Can you work these out from the model? Positions are in its coordinate system, mm. Round coordinates to 2 decimals unless told otherwise and drop trailing zeros. Write each loop counter-clockwise with the first axis right and the second up, starting at its lowest first coordinate (ties: lowest second). Pieces come first, ordered by that corner, then holes. Notation, with made-up numbers: (31, -25) -> (86, -25) arc R13 cw to (86, 0) -> close; hole circle Ø2 at (18.5, 13). An arc over 180 degrees is marked (long way). Use CSV: the item, a comma, the result in double quotes.
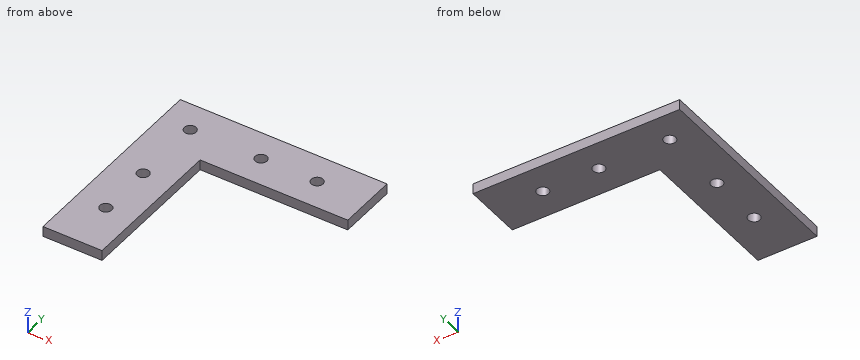
```python
from build123d import *

# Parameters (mm, degrees)
F0_R     = 2
F1_DEPTH = 3.5


with BuildPart() as f1:
    # F0 (on Top) → F1 (new body)
    with BuildSketch(Plane.XY):
        Polygon((-10, -10), (-10, -60), (10, -60), (10, -10), (60, -10), (60, 10), (10, 10), (-10, 10), align=None)
        with Locations((0, -43)):
            Circle(F0_R, mode=Mode.SUBTRACT)
        with Locations((0, -24)):
            Circle(F0_R, mode=Mode.SUBTRACT)
        Circle(F0_R, mode=Mode.SUBTRACT)
        with Locations((24, 0)):
            Circle(F0_R, mode=Mode.SUBTRACT)
        with Locations((43, 0)):
            Circle(F0_R, mode=Mode.SUBTRACT)
    extrude(amount=F1_DEPTH)


solid = f1.part
```
Q1. Suppose I cut it at A-A (y = -43). Write out the boundary of the cut face in (x, z).
Resolved:
outline,"(-10, 0) -> (-2, 0) -> (-2, 3.5) -> (-10, 3.5) -> close; (2, 0) -> (10, 0) -> (10, 3.5) -> (2, 3.5) -> close"
Q2. Suppose I cut it at C-C (z = 1.95). Write out the boundary of the cut face in (x, y).
Resolved:
outline,"(-10, -60) -> (10, -60) -> (10, -10) -> (60, -10) -> (60, 10) -> (-10, 10) -> close; hole circle Ø4 at (0, -43); hole circle Ø4 at (0, -24); hole circle Ø4 at (0, 0); hole circle Ø4 at (24, 0); hole circle Ø4 at (43, 0)"
Q3. Suppose I cut it at D-D (x = 0). Write out the boundary of the cut face in (y, z), and give its area (3 significant figures).
Resolved:
outline,"(-60, 0) -> (-45, 0) -> (-45, 3.5) -> (-60, 3.5) -> close; (-41, 0) -> (-26, 0) -> (-26, 3.5) -> (-41, 3.5) -> close; (-22, 0) -> (-2, 0) -> (-2, 3.5) -> (-22, 3.5) -> close; (2, 0) -> (10, 0) -> (10, 3.5) -> (2, 3.5) -> close"
area,"203 mm^2"
Q4. Please list where these lines run through material, in increasing order: probe 1 along Y at (x, z) = (0, 1.6); probe 2 along Y at (x, z) = (24, 2.35); probe 3 along X at (y, z) = (-46, 0.5).
Resolved:
probe 1,"y = -60 to -45, -41 to -26, -22 to -2, 2 to 10"
probe 2,"y = -10 to -2, 2 to 10"
probe 3,"x = -10 to 10"
Q5. Will these pins go through, and if not, where does the flat tip stop? P1, Ø1.5, axis at x = 21, z = 2.5, coming from the -Y side; P2, Ø3.5, axis at x = 0, y = -43, coming from the -Z side; P3, Ø1, axis at y = -32, z = 2.5, coming from the +X side.
Resolved:
P1,"stops at y = -10"
P2,"passes through"
P3,"stops at x = 10"
